Design review of the part built by this model. Coordinates are the model's own, in mm. Coordinates: 2 decimals unless noted, no trailing zeros. Write each loop counter-clockwise with the first axis right and the second up, starting at its lowest first coordinate (ties: lowest second). Pieces come first, ordered by that corner, then holes. Notation, with made-up numbers: (-23.75, 18.25) - (12.25, 18.25) arc R31 cw to (12.25, 47.25) - close; hole circle Ø7 at (74.5, -39). An arc over 180 degrees is marked (long way). Answer as CSV lines item,"result". Start each with the question number.
Q1. We need section C-C (z = -10). Write out the cut boundary in (x, y), plus the area to 3 significant figures.
Q2. Clearance check with flat-ended pins moving along their axes: pin 1 (0.5 mm diameter, centred on x = 129, y = -0.5, fed in from -Z); pin 2 (0.5 mm diameter, centred on x = 54, y = -0.5, fed in from -Z); pin 3 (8 mm diameter, centred on x = 0, z = -10, fed in from -Y). State where each tip first meets the part, or that it passes through.
Q3. We need section B-B (y = -0.75). Write out the cut boundary in (x, z).
Q4. We need section D-D (x = 60). Write out the cut boundary in (y, z).
Q5. We need section A-A (x = 0). Write out the cut boundary in (y, z).
Q6. For line 1 along Z through (x, y) = (0, -0.55); line 2 along X through (y, z) = (-0.9, 0.5); line 3 along Z through (x, y) = (32.5, -0.65), list the stretches that pass through material, from the lowest coordinate up. Write a range as [from, to].
from build123d import *

# Parameters (mm, degrees)
F0_R     = 5
F1_DEPTH = 1


with BuildPart() as f1:
    # F0 (on Front) → F1 (new body)
    with BuildSketch(Plane.XZ):
        with BuildLine():
            Line((-130, 120), (-127, 120))
            Line((-127, 120), (-127, 0))
            Line((-127, 0), (-20, 0))
            ThreePointArc((-20, 0), (0, -20), (20, 0))
            Line((20, 0), (127, 0))
            Line((127, 0), (127, 120))
            Line((127, 120), (130, 120))
            Line((130, 120), (130, 122))
            Line((130, 122), (-130, 122))
            Line((-130, 122), (-130, 120))
        make_face()
        with Locations((0, -10)):
            Circle(F0_R, mode=Mode.SUBTRACT)
    extrude(amount=F1_DEPTH)


solid = f1.part
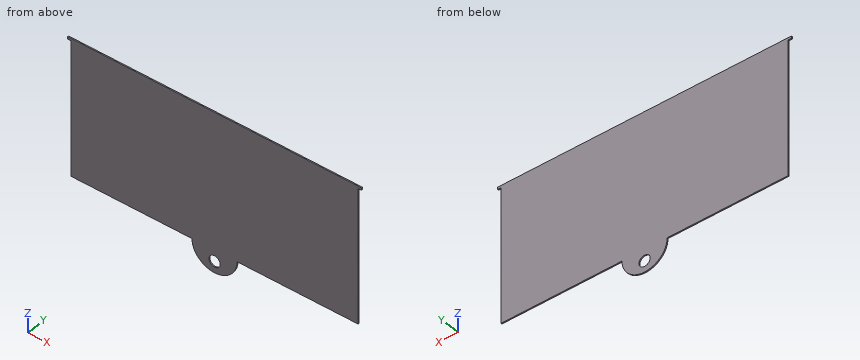
Results list:
1,outline,"(-17.32, -1) - (-5, -1) - (-5, 0) - (-17.32, 0) - close; (5, -1) - (17.32, -1) - (17.32, 0) - (5, 0) - close"
1,area,"24.6 mm2"
2,pin 1,"stops at z = 120"
2,pin 2,"stops at z = 0"
2,pin 3,"passes through"
3,outline,"(-130, 120) - (-127, 120) - (-127, 0) - (-20, 0) arc R20 ccw to (20, 0) - (127, 0) - (127, 120) - (130, 120) - (130, 122) - (-130, 122) - close; hole circle Ø10 at (0, -10)"
4,outline,"(-1, 0) - (0, 0) - (0, 122) - (-1, 122) - close"
5,outline,"(-1, -20) - (0, -20) - (0, -15) - (-1, -15) - close; (-1, -5) - (0, -5) - (0, 122) - (-1, 122) - close"
6,line 1,"z = [-20, -15], [-5, 122]"
6,line 2,"x = [-127, 127]"
6,line 3,"z = [0, 122]"
